from build123d import *

# Parameters (mm, degrees)
BASPROSKE_W              = 15
BASPROSKE_H              = 24
TOOTHCUT_DEPTH           = 38.107950631
TEETHCUTS_COUNT          = 30
TEETHCUTS_ANGLE          = 348
BORSKE_R                 = 5
BORE_DEPTH               = 50.0000508
CORTE_EXTRUS_O1_DEPTH    = 38.050491393
ESBO_O2_R                = 30.603366169
CORTE_EXTRUS_O2_DEPTH    = 5
ESBO_O4_R                = 9.5
ESBO_O4_R_2              = 7.5
RESSALTO_EXTRUS_O1_DEPTH = 1


with BuildPart() as part:
    # BasProSke → Base-Revolve (revolve)
    with BuildSketch(Plane(origin=(0, 0, 0), x_dir=(1, 0, 0), z_dir=(0, 1, 0)), mode=Mode.PRIVATE) as base_revolve_sk:
        with Locations((7.5, 12)):
            Rectangle(BASPROSKE_W, BASPROSKE_H)
    revolve(base_revolve_sk.sketch.rotate(Axis((-10, 0, 0), (1, 0, 0)), 180), axis=Axis((-10, 0, 0), (1, 0, 0)))

    # TooCutSke → ToothCut (cut, through all)
    with BuildSketch(Plane(origin=(0, 0, 0), x_dir=(0, 0, -1), z_dir=(1, 0, 0))):
        with BuildLine():
            ThreePointArc((0.693278797, 20.612344372), (0, 20.624), (-0.693278797, 20.612344372))
            ThreePointArc((-0.693278797, 20.612344372), (-1.219042225, 22.34383125), (-2.080549663, 23.935144835))
            ThreePointArc((-2.080549663, 23.935144835), (0, 24.0254), (2.080549663, 23.935144835))
            ThreePointArc((2.080549663, 23.935144835), (1.219042225, 22.34383125), (0.693278797, 20.612344372))
        make_face()
    toothcut = extrude(amount=TOOTHCUT_DEPTH, mode=Mode.SUBTRACT)

    # TeethCuts: ToothCut ×30 about axis
    teethcuts_axis = Axis((-10, 0, 0), (1, 0, 0))
    for i in range(1, TEETHCUTS_COUNT):
        add(toothcut.rotate(teethcuts_axis, i * TEETHCUTS_ANGLE / (TEETHCUTS_COUNT - 1)), mode=Mode.SUBTRACT)

    # BorSke → Bore (cut, symmetric)
    with BuildSketch(Plane(origin=(0, 0, 0), x_dir=(0, 0, -1), z_dir=(1, 0, 0))):
        with Locations(Location((0, 0, 0), (0, 0, 180))):
            Circle(BORSKE_R)
    extrude(amount=BORE_DEPTH, both=True, mode=Mode.SUBTRACT)

    # Esboço1 → Corte-extrusão1 (cut, through all)
    with BuildSketch(Plane(origin=(15, 0, 0), x_dir=(0, 0, -1), z_dir=(1, 0, 0))):
        Polygon((0, 6.5), (-5.629165125, 3.25), (-5.629165125, -3.25), (0, -6.5), (5.629165125, -3.25), (5.629165125, 3.25), align=None)
    extrude(amount=-CORTE_EXTRUS_O1_DEPTH, mode=Mode.SUBTRACT)

    # Esboço2 → Corte-extrusão2 (cut)
    with BuildSketch(Plane.ZY):
        Circle(ESBO_O2_R)
    extrude(amount=-CORTE_EXTRUS_O2_DEPTH, mode=Mode.SUBTRACT)

    # Esboço4 → Ressalto-extrusão1 (add)
    with BuildSketch(Plane.ZY.offset(-5)):
        Circle(ESBO_O4_R)
        Circle(ESBO_O4_R_2, mode=Mode.SUBTRACT)
    extrude(amount=RESSALTO_EXTRUS_O1_DEPTH)


solid = part.part
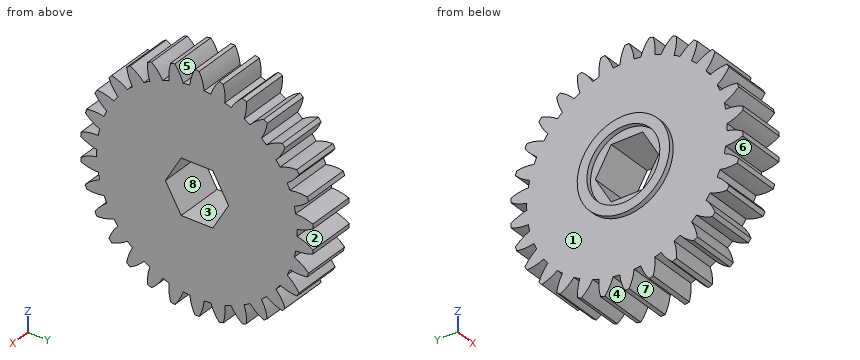
CAD build for the part. Positions are in the model's coordinates, mm. Face numbers are marked on the shaded views. A direction names the side the tool comes from. Give positions to 0.01 mm unless a question says otherwise; leave off trailing zeros. Order: outer loops, then holes, each group sorted by start corner. A loop starts at its lowest first (then second) coordinate and runs counter-clockwise, first axis right, second up. Notation, with made-up numbers: (3.5, 25.5) - (24.5, 25.5) arc R13 ccw to (24.5, 36.5) - close; hole circle Ø3 at (-39.75, 55.5). An arc over 180 degrees is marked (long way). Write each question's results on one line, items separated by ' | '.
1. Pull direction Z, two halves, no side cores. Call the marked faces 5, 6, 7 and 8: released by +Z, released by -Z, zero draft, split by the parting line, or undercut.
Calculated:
face 5: released by +Z | face 6: undercut | face 7: released by -Z | face 8: undercut
2. Pin check, flat tips, straight feed: pin 1 (3 mm diameter, centred on x = 12, y = 6, fed in from +Z); pin 2 (3 mm diameter, centred on x = 8, y = -16, fed in from +Z); pin 3 (12 mm diameter, centred on y = 2.5, z = 0, fed in from -X); pin 4 (3 mm diameter, centred on x = 6.5, z = 19, fed in from +Y). Stop position of each tip, or through.
Calculated:
pin 1: stops at z = 23.56 | pin 2: stops at z = 16.38 | pin 3: stops at x = 4 | pin 4: stops at y = 14.47
3. 3-axis set-ups, long thin cutter, end or side, ignore diameter. For the marked faces 1, 2, 3 and 4: which of +Z, -Z, +X, -X, +Y, -Y reach the whole face in a straight line?
Calculated:
face 1: -X | face 2: +X, -X, +Y | face 3: +X, -X | face 4: -Z, +X, -X
4. Saw through at A-A on z = -1.5. List the corners of the cut face in (x, y), and give its area (3 significant figures).
Calculated:
outline: (4, -9.38) - (5, -9.38) - (5, -22.95) - (15, -22.95) - (15, -5.63) - (5, -5.63) - (5, -7.35) - (4, -7.35) - close; (4, 7.35) - (5, 7.35) - (5, 5.63) - (15, 5.63) - (15, 22.95) - (5, 22.95) - (5, 9.38) - (4, 9.38) - close | area: 350 mm2
5. Probe L1, parallel to Z at x = 12, y = 22; L2, parallel to Z at x = 14, y = 18; L3, parallel to Y at x = 4.55, z = 0. List the from-to ranges inside material, lowest first. Write a range as from..to.
Calculated:
L1: z = -7.93..-6.13, -3.47..-1.08, 1.08..3.47, 6.13..7.93 | L2: z = -15.87..-15.39, -11.92..11.92, 15.39..15.87 | L3: y = -9.5..-7.5, 7.5..9.5
